Geometry check sheet. Reference: the model listing, model coordinates, mm. A direction names the side the tool comes from. Coordinates: 2 decimals unless noted, no trailing zeros. Write each loop counter-clockwise with the first axis right and the second up, starting at its lowest first coordinate (ties: lowest second). Pieces come first, ordered by that corner, then holes. Notation, with made-up numbers: (-8.5, 22.25) -> (1.5, 22.25) arc R22 cw to (1.5, 32.25) -> close; hole circle Ø1 at (-31, 22). An arc over 180 degrees is marked (long way). Put each result on its own line as item: value. Start each with the question number.
from build123d import *

# Parameters (mm, degrees)
SKETCH1_W                = 6
SKETCH1_H                = 1.2
SKETCH1_W_2              = 1.2
SKETCH1_H_2              = 4.3
REVOLVE1_ANGLE           = 180
REVOLVE2_START           = 4.3
REVOLVE2_DEPTH           = 2.7
CUT_EXTRUDE1_DEPTH       = 10
CUT_EXTRUDE2_DEPTH       = 10
SKETCH9_W                = 3.4
SKETCH9_H                = 5.5
SKETCH9_W_2              = 1.2
SKETCH9_H_2              = 3
BOSS_EXTRUDE5_DEPTH      = 2.6
SKETCH11_W               = 1.2
SKETCH11_H               = 3
CUT_EXTRUDE3_DEPTH       = 3.6
CHAMFER2_SIZE            = 0.5
CHAMFER3_SIZE            = 0.5
CHAMFER2_OF_MIRROR2_SIZE = 0.5
CHAMFER3_OF_MIRROR2_SIZE = 0.5
SKETCH5_W                = 4
SKETCH5_H                = 2
CUT_EXTRUDE4_DEPTH       = 3.6


# Read off the part's stored shape, not the designer's step: Revolve2
with BuildPart() as part:
    # Sketch1 → Revolve1 (revolve)
    with BuildSketch(Plane.XY):
        with Locations((3, -0.6)):
            Rectangle(SKETCH1_W, SKETCH1_H)
        with Locations((6.6, -0.6)):
            Rectangle(SKETCH1_W_2, SKETCH1_H)
        with Locations((6.6, 2.15)):
            Rectangle(SKETCH1_W_2, SKETCH1_H_2)
    revolve(axis=Axis((0, -1.2, 0), (0, 1, 0)), revolution_arc=REVOLVE1_ANGLE)

    # Revolve2 outline → Revolve2 (add)
    with BuildSketch(Plane(origin=(0, 0, 0), x_dir=(1, 0, 0), z_dir=(0, 1, 0)).offset(REVOLVE2_START)):
        with BuildLine():
            ThreePointArc((3.7, 6.176568627), (0, 7.2), (-3.7, 6.176568627))
            Line((-3.7, 6.176568627), (-3.7, 4.723346271))
            ThreePointArc((-3.7, 4.723346271), (0, 6), (3.7, 4.723346271))
            Line((3.7, 4.723346271), (3.7, 6.176568627))
        make_face()
    extrude(amount=REVOLVE2_DEPTH)

    # Sketch3 → Cut-Extrude1 (cut)
    with BuildSketch(Plane.XY):
        Polygon((-3.25, 1.5), (-0.75, 1.5), (-0.75, 2.5), (0.75, 2.5), (0.75, 1.5), (3.25, 1.5), (3.25, 0), (-3.25, 0), align=None)
    extrude(amount=-CUT_EXTRUDE1_DEPTH, mode=Mode.SUBTRACT)

    # Sketch4 → Cut-Extrude2 (cut)
    with BuildSketch(Plane(origin=(0, 0, 0), x_dir=(1, 0, 0), z_dir=(0, 1, 0))):
        with BuildLine():
            Line((-1.2, 0.8), (-1.2, 2.529822128))
            ThreePointArc((-1.2, 2.529822128), (-2.366431913, 1.496662955), (-2.8, 0))
            Line((-2.8, 0), (2.8, 0))
            ThreePointArc((2.8, 0), (2.366431913, 1.496662955), (1.2, 2.529822128))
            Line((1.2, 2.529822128), (1.2, 0.8))
            Line((1.2, 0.8), (-1.2, 0.8))
        make_face()
    extrude(amount=-CUT_EXTRUDE2_DEPTH, mode=Mode.SUBTRACT)

    # Sketch9 → Boss-Extrude5 (add)
    with BuildSketch(Plane(origin=(6, 0, 0), x_dir=(0, 0, -1), z_dir=(1, 0, 0))):
        with Locations((0.8, 1.55)):
            Rectangle(SKETCH9_W, SKETCH9_H)
        with Locations((0.6, 1.55)):
            Rectangle(SKETCH9_W_2, SKETCH9_H_2, mode=Mode.SUBTRACT)
    boss_extrude5 = extrude(amount=BOSS_EXTRUDE5_DEPTH)

    # Sketch11 → Cut-Extrude3 (cut)
    with BuildSketch(Plane(origin=(8.6, 0, 0), x_dir=(0, 0, -1), z_dir=(1, 0, 0))):
        with Locations((0.6, 1.55)):
            Rectangle(SKETCH11_W, SKETCH11_H)
    cut_extrude3 = extrude(amount=-CUT_EXTRUDE3_DEPTH, mode=Mode.SUBTRACT)

    # Chamfer2
    chamfer2_edges = [part.edges().sort_by_distance(p)[0] for p in [
        (8.6, 1.55, 0.9),
    ]]
    chamfer(chamfer2_edges, length=CHAMFER2_SIZE)

    # Chamfer3
    chamfer3_edges = [part.edges().sort_by_distance(p)[0] for p in [
        (8.6, 1.55, -2.5),
    ]]
    chamfer(chamfer3_edges, length=CHAMFER3_SIZE)

    # Mirror2: Boss-Extrude5, Cut-Extrude3 across plane
    add(boss_extrude5.mirror(Plane(origin=(0, 0, 0), x_dir=(0, 0, 1), z_dir=(1, 0, 0))))
    add(cut_extrude3.mirror(Plane(origin=(0, 0, 0), x_dir=(0, 0, 1), z_dir=(1, 0, 0))), mode=Mode.SUBTRACT)

    # Chamfer2 of Mirror2
    chamfer2_of_mirror2_edges = [part.edges().sort_by_distance(p)[0] for p in [
        (-8.6, 1.55, 0.9),
    ]]
    chamfer(chamfer2_of_mirror2_edges, length=CHAMFER2_OF_MIRROR2_SIZE)

    # Chamfer3 of Mirror2
    chamfer3_of_mirror2_edges = [part.edges().sort_by_distance(p)[0] for p in [
        (-8.6, 1.55, -2.5),
    ]]
    chamfer(chamfer3_of_mirror2_edges, length=CHAMFER3_OF_MIRROR2_SIZE)

    # Sketch5 → Cut-Extrude4 (cut)
    with BuildSketch(Plane(origin=(0, 0, 0), x_dir=(1, 0, 0), z_dir=(0, 1, 0))):
        with Locations((-3.6, 1)):
            Rectangle(SKETCH5_W, SKETCH5_H)
        with Locations((3.6, 1)):
            Rectangle(SKETCH5_W, SKETCH5_H)
    extrude(amount=-CUT_EXTRUDE4_DEPTH, mode=Mode.SUBTRACT)


solid = part.part
Item 1: Mould release check, pull along Z, two halves, no side actions. Record for faces 1 (the flat face through (0.75, 2, -7)), 2 (the flat face through (-7, 2, -1.2)), 3 (the flat face through (-7, 2, -2.5)), 4 (the flat face through (0, -1, -0.8)): released by +Z, released by -Z, zero draft, split by the parting line, or undercut.
Item 2: Section check B-B, the plane y = 0.25. Enter the section's corners in (x, z), and give its area (3 significant figures).
Item 3: Section check A-A, the plane x = 0. Enter the section's corners in (y, z), and give its area (3 significant figures).
Item 4: Go/stop test with flat-tipped pins: P1, Ø2, axis at x = -4.5, z = -2, coming from the +Y side; P2, Ø0.7, axis at y = 5, z = -5, coming from the -X side; P3, Ø0.8, axis at x = 8, y = 2, coming from the -Z side. Record where each tip stops, or that it passes through.
Item 5: Section check C-C, the plane z = -1.75. Enter the section's corners in (x, y).
Item 6: Section check D-D, the plane y = 3.5. Enter the section's corners in (x, z), and give its area (3 significant figures).
Item 7: Access from +Z, -Z, +X, -X, +Y, -Y to the whole of each face (thin tool, end or side, straight path). Record for faces 5 (the flat face through (7, 4.3, -2)), 6 (the flat face through (-7, 4.3, -2)), 7 (the flat face through (-7, 3.05, -1)), 8 (the flat face through (-4, -1, -2)).
Item 8: Scan lines: line 1 along Y through (x, z) = (3.25, -3.5); line 2 along Z through (x, y) = (0.75, 3.75); line 3 along Y through (x, z) = (-4, -5). Record each from-to range of solid material in increasing order. Write a range as [from, to].
From the geometry:
1. face 1: zero draft
1. face 2: undercut
1. face 3: released by -Z
1. face 4: released by +Z
2. outline: (-8.6, -2) -> (-8.1, -2.5) -> (-6.75, -2.5) arc R7.2 ccw to (-3.25, -6.42) -> (-3.25, -5.04) arc R6 cw to (-5.88, -1.2) -> (-8.6, -1.2) -> close; (-8.6, 0) -> (-6, 0) -> (-6, 0.9) -> (-8.1, 0.9) -> (-8.6, 0.4) -> close; (3.25, -6.42) arc R7.2 ccw to (6.75, -2.5) -> (8.1, -2.5) -> (8.6, -2) -> (8.6, -1.2) -> (5.88, -1.2) arc R6 cw to (3.25, -5.04) -> close; (6, 0) -> (8.6, 0) -> (8.6, 0.4) -> (8.1, 0.9) -> (6, 0.9) -> close
2. area: 22.3 mm²
3. outline: (-1.2, -7.2) -> (0, -7.2) -> (0, -0.8) -> (-1.2, -0.8) -> close; (2.5, -7.2) -> (7, -7.2) -> (7, -6) -> (2.5, -6) -> close
3. area: 13.1 mm²
4. P1: y = 0
4. P2: x = -3.7
4. P3: z = -2.5
5. outline: (-8.6, -1.2) -> (-5.6, -1.2) -> (-5.6, 0) -> (-5.74, 0) -> (-5.74, 4.3) -> (-8.6, 4.3) -> close; (-1.2, -1.2) -> (1.2, -1.2) -> (1.2, 0) -> (-1.2, 0) -> close; (5.6, -1.2) -> (8.6, -1.2) -> (8.6, 4.3) -> (5.74, 4.3) -> (5.74, 0) -> (5.6, 0) -> close
6. outline: (-8.6, -2) -> (-8.1, -2.5) -> (-6.75, -2.5) arc R7.2 ccw to (6.75, -2.5) -> (8.1, -2.5) -> (8.6, -2) -> (8.6, 0.4) -> (8.1, 0.9) -> (6, 0.9) -> (6, 0) arc R6 cw to (-6, 0) -> (-6, 0.9) -> (-8.1, 0.9) -> (-8.6, 0.4) -> close
6. area: 36.8 mm²
7. face 5: +Z, -Z, +X, +Y
7. face 6: +Z, -Z, -X, +Y
7. face 7: +X, -X
7. face 8: +Z, +Y, -Y
8. line 1: [-1.2, 0]
8. line 2: [-7.16, -5.95]
8. line 3: [-1.2, 4.3]
